Input: part model. Units: mm. Frame: model coordinates. A direction names the side the tool comes from. Give positions to 0.01 mm unless a question says otherwise; leave off trailing zeros. Loops run counter-clockwise (first coordinate to the right, second up) from the corner with the lowest first, then second, coordinate; pieces in that order, holes last. Notation, with made-up numbers: (57.25, 3) - (91.25, 3) arc R20 ccw to (91.25, 37) - close; hole circle Ø9 at (47, -2). An arc over 180 degrees is marked (long way). Answer as a JSON object with one key per item and string values. Group by question number.
(1) Section query B-B (x = -45.5). Return loops of the section in (y, z).
(2) Section query A-A (z = 44.5). Return loops of the section in (x, y).
(3) Section query D-D (x = 10.5). Return loops of the section in (y, z), plus the area to 3 significant figures.
(4) Material intervals for L1, parallel to Y at x = 43.5, z = 5.5; L2, parallel to Z at x = -2, y = -27; L3, parallel to X at y = -17.5, z = -3, sorted ascending.
(5) Access query for faces 4 (the flat face through (-27, 0, 20)), 5 (the flat face through (-24.891, -38, 22)). Directions: +Z, -Z, +X, -X, +Y, -Y. A direction counts if a zero-diameter tool reaches every point of the face in a straight line with its end or side. Return the directions, or none.
(6) Mould query, pull axis Z, two halves, no side actions, for faces 1 (the flat face through (-45, -50.8, 20)), 2 (the cylindrical face through (-53.044, -25.044, 29.617)), 3 (the flat face through (8.456, -12.522, 31.851)). Classes: +Z half, -Z half, draft (parallel to the pull), parting line (faces both ways), or undercut.
(7) Pin query (flat end, axial travel): P1, Ø5, axis at x = -12.5, z = 33, coming from the -Y side; P2, Ø3, axis at y = -25, z = 4, coming from the +X side; P3, Ø20.5, axis at y = -37, z = 18.5, coming from the +X side. Return the tip coordinate at first contact, or that it passes through.
(8) Section query C-C (y = -5). Return loops of the section in (x, z), plus the area to 3 significant figures.
```python
from build123d import *

# Parameters (mm, degrees)
F0_R     = 12.7
F1_DEPTH = 25.4
F2_R     = 12.7
F3_DEPTH = 25.4
F4_R     = 12.7


with BuildPart() as f1:
    # F0 (on Front) → F1 (new body)
    with BuildSketch(Plane.XZ):
        with BuildLine():
            ThreePointArc((-75.5979648529, 39.8426862847), (-49.2037324517, 16.6386265616), (-24.8910574185, 42.0153427482))
            ThreePointArc((-24.8910574185, 42.0153427482), (-27.7576393347, 53.737333597), (-35.7103542263, 62.8134939742))
            ThreePointArc((-35.7103542263, 62.8134939742), (-62.9669150163, 64.0263089733), (-75.5979648529, 39.8426862847))
        make_face()
        with Locations((-50.2910574185, 42.0153427482)):
            Circle(F0_R, mode=Mode.SUBTRACT)
        with BuildLine():
            ThreePointArc((-35.7103542263, 62.8134939742), (-27.7576393347, 53.737333597), (-24.8910574185, 42.0153427482))
            ThreePointArc((-24.8910574185, 42.0153427482), (-49.2037324517, 16.6386265616), (-75.5979648529, 39.8426862847))
            Line((-75.5979648529, 39.8426862847), (-75.5979648529, -10.9573137153))
            Line((-75.5979648529, -10.9573137153), (51.4020351471, -10.9573137153))
            Line((51.4020351471, -10.9573137153), (51.4020351471, 1.7426862847))
            Line((51.4020351471, 1.7426862847), (-35.7103542263, 62.8134939742))
        make_face()
    extrude(amount=F1_DEPTH)

    # F2 (on face) → F3 (join)
    with BuildSketch(Plane.XZ.offset(25.4)):
        with BuildLine():
            Line((-24.8910574185, 1.7426862847), (-24.8910574185, 42.0153427482))
            ThreePointArc((-24.8910574185, 42.0153427482), (-27.7576393347, 53.737333597), (-35.7103542263, 62.8134939742))
            ThreePointArc((-35.7103542263, 62.8134939742), (-62.0130482673, 64.548760832), (-75.6910574185, 42.0153427482))
            ThreePointArc((-75.6910574185, 42.0153427482), (-75.6909895589, 41.9566293417), (-75.6907859804, 41.8979162489))
            ThreePointArc((-75.6907859804, 41.8979162489), (-75.6651924002, 40.8693611015), (-75.5979648529, 39.8426862847))
            Line((-75.5979648529, 39.8426862847), (-75.5979648529, 1.7426862847))
            Line((-75.5979648529, 1.7426862847), (-75.5979648529, -10.9573137153))
            Line((-75.5979648529, -10.9573137153), (51.4020351471, -10.9573137153))
            Line((51.4020351471, -10.9573137153), (51.4020351471, 1.7426862847))
            Line((51.4020351471, 1.7426862847), (-24.8910574185, 1.7426862847))
        make_face()
        with Locations((-50.2910574185, 42.0153427482)):
            Circle(F2_R, mode=Mode.SUBTRACT)
    extrude(amount=F3_DEPTH)

    # F4
    f4_edges = [f1.edges().sort_by_distance(p)[0] for p in [
        (51.402035, -50.8, -4.607314),
    ]]
    fillet(f4_edges, radius=F4_R)


solid = f1.part
```
Recorded:
{
 "1": {"outline": "(-50.8, -10.96) - (0, -10.96) - (0, 30.25) - (-50.8, 30.25) - close; (-50.8, 53.78) - (0, 53.78) - (0, 66.96) - (-50.8, 66.96) - close"},
 "2": {"outline": "(-75.57, -50.8) - (-62.75, -50.8) - (-62.75, 0) - (-75.57, 0) - close; (-37.84, -50.8) - (-25.01, -50.8) - (-25.01, -25.4) - (-9.59, -25.4) - (-9.59, 0) - (-37.84, 0) - close"},
 "3": {"outline": "(-50.8, -10.96) - (0, -10.96) - (0, 30.42) - (-25.4, 30.42) - (-25.4, 1.74) - (-50.8, 1.74) - close", "area": "1,370 mm^2"},
 "4": {"L1": "y = -25.4 to 0", "L2": "z = -10.96 to 1.74", "L3": "x = -75.6 to 51.4"},
 "5": {"face 4": "+Z, -Z, +X, -X, +Y", "face 5": "+Z, +X, -Y"},
 "6": {"face 1": "draft", "face 2": "undercut", "face 3": "+Z half"},
 "7": {"P1": "stops at y = -25.4", "P2": "stops at x = 50.32", "P3": "stops at x = -24.89"},
 "8": {"outline": "(-75.6, -10.96) - (51.4, -10.96) - (51.4, 1.74) - (-35.71, 62.81) arc R25.4 ccw to (-75.6, 39.84) - close; hole circle Ø25.4 at (-50.29, 42.02)", "area": "6,230 mm^2"}
}
